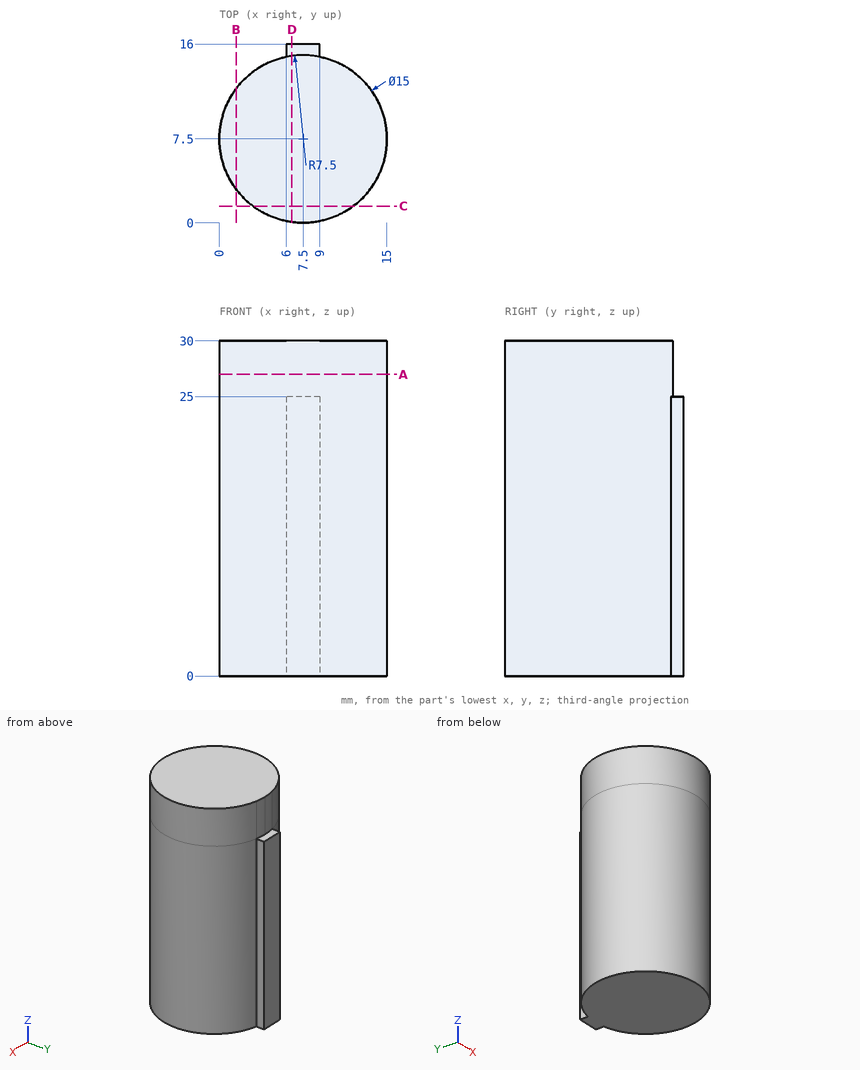
Could you check a few things on this drawing? It's one solid part, dimensions in mm from its lowest x, y, z. Coordinates: 2 decimals unless noted, no trailing zeros. Order: outer loops, then holes, each group sorted by start corner. A loop starts at its lowest first (then second) coordinate and runs counter-clockwise, first axis right, second up. Notation, with made-up numbers: M 42.25,77.25 L 63.25,77.25 A13 cw 63.25,98.25 Z; hole C 70,0 d10. An arc over 180 degrees is marked long. Answer as CSV lines item,"result".
(1) Suppose I cut it at D-D on x = 6.5. Please give me the cut outline in (y, z), plus the area to 3 significant figures.
Geometry check:
outline,"M 0.07,0 L 16,0 L 16,25 L 14.93,25 L 14.93,30 L 0.07,30 Z"
area,"473 mm^2"
(2) Suppose I cut it at A-A on z = 27. Please give me the cut outline in (x, y).
Geometry check:
outline,"C 7.5,7.5 d15"
(3) Suppose I cut it at B-B on x = 1.5. Please give me the cut outline in (y, z), plus the area to 3 significant figures.
Geometry check:
outline,"M 3,0 L 12,0 L 12,30 L 3,30 Z"
area,"270 mm^2"
(4) Please list where these lines run through material, in increasing order: L1, parallel to X at y = 11.5, z = 23; L2, parallel to X at y = 15.25, z = 17.75; L3, parallel to Y at x = 10.25, z = 21.
Geometry check:
L1,"1.16 to 13.84"
L2,"6 to 9"
L3,"0.52 to 14.48"
(5) I'm going to push flat-ended pins straight in: pin 1 (0.9 mm diameter, centred on x = 7, y = 15.5, fed in from +Z); pin 2 (1 mm diameter, centred on x = 5, z = 27, fed in from +Y); pin 3 (5 mm diameter, centred on y = 4, z = 14, fed in from -X). Where does each tip first touch, or does it pass through?
Geometry check:
pin 1,"z = 25"
pin 2,"y = 14.73"
pin 3,"x = 0.07"
